Verification items for this drawing (mm, ordinates from the low corner). A direction names the side the tool comes from. Round coordinates to 2 decimals unless told otherwise and drop trailing zeros. Order: outer loops, then holes, each group sorted by start corner. A loop starts at its lowest first (then second) coordinate and runs counter-clockwise, first axis right, second up.
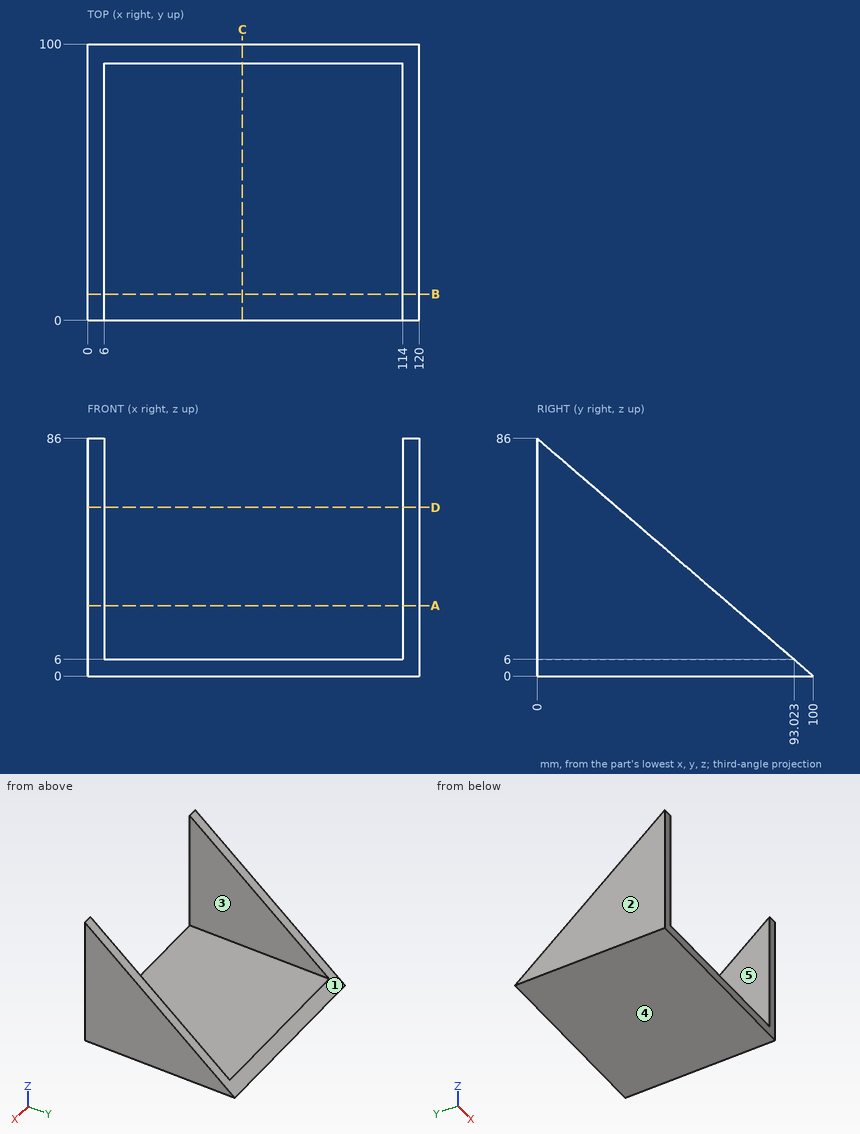
Item 1: Access from +Z, -Z, +X, -X, +Y, -Y to the whole of each face (thin tool, end or side, straight path). Record for the marked faces 4 and 5.
Answer:
face 4: -Z, +X, -X, +Y, -Y
face 5: +Z, +Y, -Y
Item 2: Sectioned sample at B-B (y = 9.5). Record the cut outline in (x, z), and give its area (3 significant figures).
Answer:
outline: (0, 0) - (120, 0) - (120, 77.83) - (114, 77.83) - (114, 6) - (6, 6) - (6, 77.83) - (0, 77.83) - close
area: 1,580 mm2
Item 3: Go/stop test with a flat-tipped pin: P1, Ø24, axis at y = 68, z = 52.5, coming from the -X side. Record where the tip stops, or that it passes through.
Answer:
P1: passes through
Item 4: Sectioned sample at A-A (z = 25.5). Record the cut outline in (x, y).
Answer:
outline: (0, 0) - (6, 0) - (6, 70.35) - (0, 70.35) - close; (114, 0) - (120, 0) - (120, 70.35) - (114, 70.35) - close
Item 5: Release check for a two-part mould opening along X. For the marked faces 1, 2 and 3 record: released by +X, released by -X, zero draft, split by the parting line, or undercut.
Answer:
face 1: zero draft
face 2: released by -X
face 3: undercut
Item 6: Scan lines: line 1 along X through (y, z) = (41.5, 38); line 2 along Z through (x, y) = (74, 26.5); line 3 along Z through (x, y) = (114.5, 83.5). Record each from-to range of solid material in increasing order.
Answer:
line 1: x = 0 to 6, 114 to 120
line 2: z = 0 to 6
line 3: z = 0 to 14.19
Item 7: Sectioned sample at C-C (x = 56). Record the cut outline in (y, z), and give its area (3 significant figures).
Answer:
outline: (0, 0) - (100, 0) - (93.02, 6) - (0, 6) - close
area: 579 mm2
Item 8: Sectioned sample at D-D (z = 61). Record the cut outline in (x, y), and give its area (3 significant figures).
Answer:
outline: (0, 0) - (6, 0) - (6, 29.07) - (0, 29.07) - close; (114, 0) - (120, 0) - (120, 29.07) - (114, 29.07) - close
area: 349 mm2
